```python
from build123d import *

# Parameters (mm, degrees)
SCHIZZO1_W                   = 83.5
SCHIZZO1_H                   = 83.5
ESTRUSIONE_ESTRUSIONE1_DEPTH = 3
SCHIZZO2_R                   = 2
TAGLIO_ESTRUSIONE1_DEPTH     = 3
TAGLIO_ESTRUSIONE2_DEPTH     = 60.119582204
RIPETIZIONE_A_L1_COUNT       = 2
RIPETIZIONE_A_L1_PITCH       = 51
RIPETIZIONE_A_L1_COUNT_DIR2  = 2
RIPETIZIONE_A_L1_PITCH_DIR2  = 25
SPECCHIA1_COPY_1_DEPTH       = 60.119582204
SPECCHIA1_COPY_2_DEPTH       = 60.119582204
SPECCHIA1_COPY_3_DEPTH       = 60.119582204
SPECCHIA1_COPY_4_DEPTH       = 60.119582204


with BuildPart() as part:
    # Schizzo1 → Estrusione-Estrusione1 (new body)
    with BuildSketch(Plane(origin=(0, 0, 0), x_dir=(1, 0, 0), z_dir=(0, 1, 0))):
        Rectangle(SCHIZZO1_W, SCHIZZO1_H)
    extrude(amount=ESTRUSIONE_ESTRUSIONE1_DEPTH)

    # Schizzo2 → Taglio-Estrusione1 (cut)
    with BuildSketch(Plane(origin=(0, 0, 0), x_dir=(-1, 0, 0), z_dir=(0, -1, 0))):
        with Locations(Location((39.621320344, 39.621320344, 0), (0, 0, 90))):
            Circle(SCHIZZO2_R)
        with Locations(Location((39.621320344, -39.621320344, 0), (0, 0, 90))):
            Circle(SCHIZZO2_R)
        with Locations(Location((-39.621320344, 39.621320344, 0), (0, 0, 90))):
            Circle(SCHIZZO2_R)
        with Locations(Location((-39.621320344, -39.621320344, 0), (0, 0, 90))):
            Circle(SCHIZZO2_R)
    extrude(amount=-TAGLIO_ESTRUSIONE1_DEPTH, mode=Mode.SUBTRACT)

    # Schizzo4 → Taglio-Estrusione2 (cut, through all)
    with BuildSketch(Plane.XZ):
        with BuildLine():
            Line((-27.75, 1.75), (-31.75, 1.75))
            ThreePointArc((-31.75, 1.75), (-33.5, 0), (-31.75, -1.75))
            Line((-31.75, -1.75), (-27.75, -1.75))
            Line((-27.75, -1.75), (-23.347020102, -3.667359649))
            ThreePointArc((-23.347020102, -3.667359649), (-17.75, 0), (-23.347020102, 3.667359649))
            Line((-23.347020102, 3.667359649), (-27.75, 1.75))
        make_face()
    taglio_estrusione2 = extrude(amount=-TAGLIO_ESTRUSIONE2_DEPTH, mode=Mode.SUBTRACT)

    # Ripetizione a L1: Taglio-Estrusione2 2 × 2
    with Locations(*[(i * RIPETIZIONE_A_L1_PITCH, 0, -j * RIPETIZIONE_A_L1_PITCH_DIR2) for i in range(RIPETIZIONE_A_L1_COUNT) for j in range(RIPETIZIONE_A_L1_COUNT_DIR2) if (i, j) != (0, 0)]):
        add(taglio_estrusione2, mode=Mode.SUBTRACT)

    # Specchia1 copy 1 sketch → Specchia1 copy 1 (cut, through all)
    with BuildSketch(Plane(origin=(0, 0, 25), x_dir=(1, 0, 0), z_dir=(0, -1, 0))):
        with BuildLine():
            Line((-27.75, -1.75), (-31.75, -1.75))
            ThreePointArc((-31.75, -1.75), (-33.5, 0), (-31.75, 1.75))
            Line((-31.75, 1.75), (-27.75, 1.75))
            Line((-27.75, 1.75), (-23.347020102, 3.667359649))
            ThreePointArc((-23.347020102, 3.667359649), (-17.75, 0), (-23.347020102, -3.667359649))
            Line((-23.347020102, -3.667359649), (-27.75, -1.75))
        make_face()
    extrude(amount=-SPECCHIA1_COPY_1_DEPTH, mode=Mode.SUBTRACT)

    # Specchia1 copy 2 sketch → Specchia1 copy 2 (cut, through all)
    with BuildSketch(Plane(origin=(51, 0, 0), x_dir=(1, 0, 0), z_dir=(0, -1, 0))):
        with BuildLine():
            Line((-27.75, -1.75), (-31.75, -1.75))
            ThreePointArc((-31.75, -1.75), (-33.5, 0), (-31.75, 1.75))
            Line((-31.75, 1.75), (-27.75, 1.75))
            Line((-27.75, 1.75), (-23.347020102, 3.667359649))
            ThreePointArc((-23.347020102, 3.667359649), (-17.75, 0), (-23.347020102, -3.667359649))
            Line((-23.347020102, -3.667359649), (-27.75, -1.75))
        make_face()
    extrude(amount=-SPECCHIA1_COPY_2_DEPTH, mode=Mode.SUBTRACT)

    # Specchia1 copy 3 sketch → Specchia1 copy 3 (cut, through all)
    with BuildSketch(Plane(origin=(51, 0, 25), x_dir=(1, 0, 0), z_dir=(0, -1, 0))):
        with BuildLine():
            Line((-27.75, -1.75), (-31.75, -1.75))
            ThreePointArc((-31.75, -1.75), (-33.5, 0), (-31.75, 1.75))
            Line((-31.75, 1.75), (-27.75, 1.75))
            Line((-27.75, 1.75), (-23.347020102, 3.667359649))
            ThreePointArc((-23.347020102, 3.667359649), (-17.75, 0), (-23.347020102, -3.667359649))
            Line((-23.347020102, -3.667359649), (-27.75, -1.75))
        make_face()
    extrude(amount=-SPECCHIA1_COPY_3_DEPTH, mode=Mode.SUBTRACT)

    # Specchia1 copy 4 sketch → Specchia1 copy 4 (cut, through all)
    with BuildSketch(Plane.XZ):
        with BuildLine():
            Line((-27.75, -1.75), (-31.75, -1.75))
            ThreePointArc((-31.75, -1.75), (-33.5, 0), (-31.75, 1.75))
            Line((-31.75, 1.75), (-27.75, 1.75))
            Line((-27.75, 1.75), (-23.347020102, 3.667359649))
            ThreePointArc((-23.347020102, 3.667359649), (-17.75, 0), (-23.347020102, -3.667359649))
            Line((-23.347020102, -3.667359649), (-27.75, -1.75))
        make_face()
    extrude(amount=-SPECCHIA1_COPY_4_DEPTH, mode=Mode.SUBTRACT)


solid = part.part
```
For this review, take the finished solid that the model builds, in its own axes (mm). A direction names the side the tool comes from. Coordinates: 2 decimals unless noted, no trailing zeros. Loops run counter-clockwise (first coordinate to the right, second up) from the corner with the lowest first, then second, coordinate; pieces in that order, holes last. Notation, with made-up numbers: (-18.75, -1) - (3.25, -1) arc R22 ccw to (3.25, 15) - close; hole circle Ø10 at (31.25, 23). An arc over 180 degrees is marked (long way). Use one line per item in the form item = value. Start each with the question number.
1) To check wall thickness, follow probe 1 along X at (y, z) = (1.75, 25); probe 2 along Z at (x, y) = (-22, 2.85); probe 3 along Z at (x, y) = (19, 1.35). State the ranges of each line that lie inside material, in increasing order. Write a range as from..to.
2) Take a section at D-D (y = 1.85). State how many separate pieces and enclosed holes the cut face has, plus the area to 3 significant figures.
3) Take a section at B-B (x = 29.25). State the section outline as (y, z) points.
4) For pin 1 (3.5 mm diameter, centred on x = 39.62, z = 39.62, fed in from +Y), flat-tipped, find the tip position at first contact; note if it passes through.
5) Take a section at A-A (z = 0). State the section outline as (x, y) points, plus the area to 3 significant figures.
6) Draft analysis for pull direction X (two halves, no side actions). For faces 3 (the face through (-1, 1, -41.75)), 4 (the face through (-25.579, 1.479, -2.695)), 5 (the face through (-41.75, 1, 1)), state which applies: released by +X, released by -X, zero draft, split by the parting line, or undercut.
7) For faces 1 (the face through (-1, 3, -1)), 2 (the face through (25.48, 1.48, -22.28)), list the 3-axis set-ups (+Z, -Z, +X, -X, +Y, -Y) from which the entire face can be reached by the end or side of a thin tool; tool diameter is ignored.
8) Take a section at C-C (x = -24.5). State the section outline as (y, z) points, plus the area to 3 significant figures.
From the geometry:
q1.probe_1 = -41.75..-33.5, -17.75..17.5, 33.25..41.75
q1.probe_2 = -41.75..-28.99, -21.01..-3.99, 3.99..21.01, 28.99..41.75
q1.probe_3 = -41.75..-26.73, -23.27..-1.73, 1.73..23.27, 26.73..41.75
q2.separate_pieces = 1
q2.enclosed_holes = 10
q2.area = 6,440 mm2
q3.outline = (0, -41.75) - (3, -41.75) - (3, -29) - (0, -29) - close; (0, -21) - (3, -21) - (3, -4) - (0, -4) - close; (0, 4) - (3, 4) - (3, 21) - (0, 21) - close; (0, 29) - (3, 29) - (3, 41.75) - (0, 41.75) - close
q4.pin_1 = through
q5.outline = (-41.75, 0) - (-33.5, 0) - (-33.5, 3) - (-41.75, 3) - close; (-17.75, 0) - (17.5, 0) - (17.5, 3) - (-17.75, 3) - close; (33.25, 0) - (41.75, 0) - (41.75, 3) - (33.25, 3) - close
q5.area = 156 mm2
q6.face_3 = zero draft
q6.face_4 = undercut
q6.face_5 = released by -X
q7.face_1 = +Z, -Z, +X, -X, +Y
q7.face_2 = +Y, -Y
q8.outline = (0, -41.75) - (3, -41.75) - (3, -28.17) - (0, -28.17) - close; (0, -21.83) - (3, -21.83) - (3, -3.17) - (0, -3.17) - close; (0, 3.17) - (3, 3.17) - (3, 21.83) - (0, 21.83) - close; (0, 28.17) - (3, 28.17) - (3, 41.75) - (0, 41.75) - close
q8.area = 194 mm2
